Source: CAD feature listing. Evaluate the final solid. Frame: model axes, mm. A direction names the side the tool comes from. Give positions to 0.01 mm unless a question says otherwise; leave off trailing zeros. Order: outer loops, then holes, each group sorted by start corner. A loop starts at its lowest first (then second) coordinate and runs counter-clockwise, first axis right, second up. Notation, with made-up numbers: (2, 48) - (6, 48) arc R19 ccw to (6, 52) - close; hole circle Ø10 at (41.25, -23). An arc over 180 degrees is marked (long way). Write each question's results on one line, items separated by ' | '. Start each with the question number.
Item 1: Section A-A on y = 1.25. Output: boundary loops of the cut face in (x, z).
Item 2: Section C-C on y = 24. Output: boundary loops of the cut face in (x, z) (3 decimals).
Item 3: Set-up query: faces 4 (the flat face through (10.4, 2.5, -10.4)), 5 (the flat face through (0, -1, 0)), 6 (the cylindrical face through (-0.9, -0.49, 2.86)). Return all of +Z, -Z, +X, -X, +Y, -Y with unobstructed straight access to the full face (end or side cutting, diameter ignored); none if empty.
Item 4: Mould query, pull axis Z, two halves, no side actions, for faces 1 (the cylindrical face through (-10.75, 1.52, -0.05)), 2 (the cylindrical face through (-0.065, 23.512, 1.474)), 3 (the flat face through (6.746, 0.955, -12.403)). Classes: released by +Z, released by -Z, zero draft, split by the parting line, or undercut.
Item 5: Contact query for flat-ended pins moving along their axis: pin 1 Ø4 at (x, z) = (9.5, -11.5) entering from +Y; pin 2 Ø3 at (x, z) = (-9.5, 0) entering from +Y; pin 3 Ø8 at (x, y) = (4.5, 19.5) entering from +Z; pin 4 Ø2 at (x, y) = (3.5, 22.5) entering from +Z (3 decimals). Output: stop coordinate, or through.
Item 6: Section B-B on y = 17.5. Output: boundary loops of the cut face in (x, z), and give its area (3 significant figures).
Item 7: Line query: line 1 along Z through (x, y) = (0, 1.85); line 2 along Y through (x, z) = (-4.25, 0); line 3 along X through (y, z) = (1.7, 8). Output: solid intervals per line, ascending.
```python
from build123d import *

# Parameters (mm, degrees)
SKIZZE1_R                  = 14.5
GRUNDKOERPER_DEPTH         = 19
GRUNDKOERPERFASE_SIZE      = 2.5
MONTAGEBOHRUNG_UNTEN_D     = 2.5
MONTAGEBOHRUNG_UNTEN_DEPTH = 3
MONTAGEBOHRUNG_UNTEN_TIP   = 0.751075774
SKIZZE6_W                  = 1.475
SKIZZE6_H                  = 9.2
AUFNAHME_FASE_SIZE         = 0.3
SKIZZE7_R                  = 3
WELLENUEBERSTAND_DEPTH     = 1
SKIZZE8_W                  = 2.5
SKIZZE8_H                  = 8
KABELANSCHLUSS_DEPTH       = 5


with BuildPart() as part:
    # Skizze1 → Grundkoerper (new body)
    with BuildSketch(Plane(origin=(0, 0, 0), x_dir=(1, 0, 0), z_dir=(0, 1, 0))):
        with Locations(Location((0, 0, 0), (0, 0, 270))):
            Circle(SKIZZE1_R)
    extrude(amount=GRUNDKOERPER_DEPTH)

    # Grundkoerperfase
    grundkoerperfase_edges = [part.edges().sort_by_distance(p)[0] for p in [
        (0, 0, -14.5),
        (0, 19, -14.5),
    ]]
    chamfer(grundkoerperfase_edges, length=GRUNDKOERPERFASE_SIZE)

    # Montagebohrung unten
    with Locations(Plane(origin=(0, 0, 0), x_dir=(-1, 0, 0), z_dir=(0, -1, 0))):
        with Locations((9.5, 0), (0, -8), (-9.5, 0), (0, 8)):
            Hole(MONTAGEBOHRUNG_UNTEN_D / 2, depth=MONTAGEBOHRUNG_UNTEN_DEPTH)
            with Locations((0, 0, -(MONTAGEBOHRUNG_UNTEN_DEPTH + MONTAGEBOHRUNG_UNTEN_TIP / 2))):  # 118° drill point
                Cone(0, MONTAGEBOHRUNG_UNTEN_D / 2, MONTAGEBOHRUNG_UNTEN_TIP, mode=Mode.SUBTRACT)

    # Skizze6 → Propelleraufnahme (revolve)
    with BuildSketch(Plane.XY, mode=Mode.PRIVATE) as propelleraufnahme_sk:
        with Locations((0.7375, 23.6)):
            Rectangle(SKIZZE6_W, SKIZZE6_H)
    revolve(propelleraufnahme_sk.sketch.rotate(Axis((0, -3.27786324, 0), (0, 1, 0)), 90), axis=Axis((0, -3.27786324, 0), (0, 1, 0)))

    # Aufnahme_Fase
    aufnahme_fase_edges = [part.edges().sort_by_distance(p)[0] for p in [
        (0, 28.2, 1.475),
    ]]
    chamfer(aufnahme_fase_edges, length=AUFNAHME_FASE_SIZE)

    # Skizze7 → Wellenueberstand (add)
    with BuildSketch(Plane.XZ):
        with Locations(Location((0, 0, 0), (0, 0, 90))):
            Circle(SKIZZE7_R)
    extrude(amount=WELLENUEBERSTAND_DEPTH)

    # Skizze8 → Kabelanschluss (add)
    with BuildSketch(Plane(origin=(7.071067812, 0, -7.071067812), x_dir=(0, 1, 0), z_dir=(-0.7071067811865488, 0, 0.7071067811865464))):
        with Locations((1.25, 0)):
            Rectangle(SKIZZE8_W, SKIZZE8_H)
    extrude(amount=-KABELANSCHLUSS_DEPTH)


solid = part.part
```
Evaluation:
1) outline: (6.1, -11.76) - (7.78, -13.44) - (13.44, -7.78) - (11.76, -6.1) arc R13.25 ccw (long way) to start; hole circle Ø2.5 at (-9.5, 0); hole circle Ø2.5 at (0, -8); hole circle Ø2.5 at (0, 8); hole circle Ø2.5 at (9.5, 0)
2) outline: circle Ø2.95 at (0, 0)
3) face 4: -Z, +X, +Y | face 5: +Z, -Z, +X, -X, -Y | face 6: -Y
4) face 1: undercut | face 2: split by the parting line | face 3: released by -Z
5) pin 1: stops at y = 18.08 | pin 2: stops at y = 19 | pin 3: stops at z = 14.38 | pin 4: passes through
6) outline: circle Ø27 at (0, 0) | area: 573 mm^2
7) line 1: z = -13.85 to -9.25, -6.75 to 6.75, 9.25 to 13.85 | line 2: y = 0 to 19 | line 3: x = -11.12 to -1.25, 1.25 to 11.12
